CAD build for the part. Positions are in the model's coordinates, mm. Give positions to 0.01 mm unless a question says otherwise; leave off trailing zeros. Write each loop counter-clockwise with the first axis right and the second up, starting at its lowest first coordinate (ties: lowest second). Pieces come first, ordered by that corner, then holes. Notation, with made-up numbers: (19.5, 77.5) - (60.5, 77.5) arc R9 ccw to (60.5, 84.5) - close; hole circle Ø11 at (-21, -25). An arc over 180 degrees is marked (long way). Answer as a JSON object with one key per item and string values.
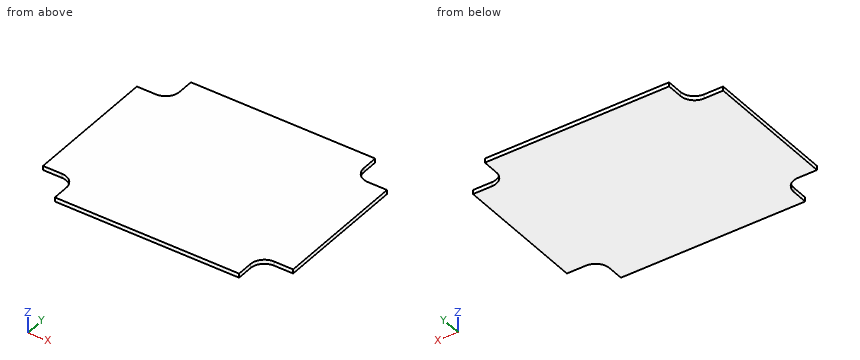
from build123d import *

# Parameters (mm, degrees)
SKETCH_3_W      = 66.3
SKETCH_3_H      = 48.3
SKETCH_3_W_2    = 11.85
SKETCH_3_H_2    = 10.85
EXTRUDE_1_DEPTH = 1.5
FILLET_1_R      = 5


with BuildPart() as part:
    # 草图3 → 凸台-拉伸1 (new body)
    with BuildSketch(Plane.XY):
        with Locations((-0.073737011, -0.836272376)):
            Rectangle(SKETCH_3_W, SKETCH_3_H)
        with Locations((-39.148737011, -0.836272376)):
            Rectangle(SKETCH_3_W_2, SKETCH_3_H)
        with Locations((-0.073737011, -30.411272376)):
            Rectangle(SKETCH_3_W, SKETCH_3_H_2)
        with Locations((-0.073737011, 28.738727624)):
            Rectangle(SKETCH_3_W, SKETCH_3_H_2)
        with Locations((39.001262989, -0.836272376)):
            Rectangle(SKETCH_3_W_2, SKETCH_3_H)
    extrude(amount=EXTRUDE_1_DEPTH)

    # 圆角1
    fillet_1_edges = [part.edges().sort_by_distance(p)[0] for p in [
        (33.076262989, 23.313727624, 0.75),
        (33.076262989, -24.986272376, 0.75),
        (-33.223737011, -24.986272376, 0.75),
        (-33.223737011, 23.313727624, 0.75),
    ]]
    fillet(fillet_1_edges, radius=FILLET_1_R)


solid = part.part
Item 1: Cut at A-A (z = 0.4). Give the cut face in (x, y), and give its area (3 significant figures).
Entries:
{"outline": "(-45.07, -24.99) - (-38.22, -24.99) arc R5 cw to (-33.22, -29.99) - (-33.22, -35.84) - (33.08, -35.84) - (33.08, -29.99) arc R5 cw to (38.08, -24.99) - (44.93, -24.99) - (44.93, 23.31) - (38.08, 23.31) arc R5 cw to (33.08, 28.31) - (33.08, 34.16) - (-33.22, 34.16) - (-33.22, 28.31) arc R5 cw to (-38.22, 23.31) - (-45.07, 23.31) - close", "area": "5,810 mm2"}
Item 2: Flat gauge pins, fed straight in: P1, Ø0.8, axis at y = -32, z = 1, coming from the -X side; P2, Ø0.8, axis at x = -42, z = 0.5, coming from the -Y side. Where does each tip first touch, or does it go through?
Entries:
{"P1": "x = -33.22", "P2": "y = -24.99"}
Item 3: Probe line 1 (X direction, y = -30.5, z = 0.7); line 2 (X direction, y = 25, z = 1.3); line 3 (Y direction, x = 37, z = 1.3). List the from-to ranges inside material, lowest first. Write a range as from..to.
Entries:
{"line 1": "-33.22..33.08", "line 2": "-34.48..34.33", "line 3": "-25.1..23.43"}
Item 4: Cut at C-C (x = 36.5). Give the cut face in (y, z).
Entries:
{"outline": "(-25.24, 0) - (23.57, 0) - (23.57, 1.5) - (-25.24, 1.5) - close"}
Item 5: Cut at B-B (y = 30). Give the cut face in (x, z), and give its area (4 significant figures).
Entries:
{"outline": "(-33.22, 0) - (33.08, 0) - (33.08, 1.5) - (-33.22, 1.5) - close", "area": "99.45 mm2"}
